from build123d import *

# Parameters (mm, degrees)
BOSS_EXTRUDE1_DEPTH = 64.15
SKETCH2_R           = 1.75
CUT_EXTRUDE1_DEPTH  = 2.42
CUT_EXTRUDE2_DEPTH  = 2.42
SKETCH4_R           = 1.54
CUT_EXTRUDE3_DEPTH  = 2.42


with BuildPart() as part:
    # Sketch1 → Boss-Extrude1 (new, symmetric)
    with BuildSketch(Plane(origin=(0, 0, 0), x_dir=(0, 0, -1), z_dir=(1, 0, 0))):
        with BuildLine():
            Line((-22.947001366, 0), (-3.987001366, 0))
            ThreePointArc((-3.987001366, 0), (-1.844787094, 1.175258995), (-1.684979587, 3.613450385))
            Line((-1.684979587, 3.613450385), (-7.115854863, 15.26))
            Line((-7.115854863, 15.26), (-9.309119708, 14.237263807))
            Line((-9.309119708, 14.237263807), (-3.878244431, 2.590714191))
            ThreePointArc((-3.878244431, 2.590714191), (-3.885794392, 2.475524047), (-3.987001366, 2.42))
            Line((-3.987001366, 2.42), (-22.947001366, 2.42))
            Line((-22.947001366, 2.42), (-22.947001366, 0))
        make_face()
    extrude(amount=BOSS_EXTRUDE1_DEPTH, both=True)

    # Sketch2 → Cut-Extrude1 (cut)
    with BuildSketch(Plane(origin=(0, 0, 0), x_dir=(-1, 0, 0), z_dir=(0, 0.4226182617407038, -0.9063077870366478))):
        with BuildLine():
            ThreePointArc((-64.15, 11.687547043), (-62.641599916, 15.329146974), (-58.999999979, 16.837547043))
            Line((-58.999999979, 16.837547043), (-64.15, 16.837547043))
            Line((-64.15, 16.837547043), (-64.15, 11.687547043))
        make_face()
        with BuildLine():
            ThreePointArc((54.05757399, 13.134932664), (55.912244813, 15.809229698), (58.999999973, 16.837547043))
            Line((58.999999973, 16.837547043), (-58.999999979, 16.837547043))
            ThreePointArc((-58.999999979, 16.837547043), (-55.912244816, 15.8092297), (-54.05757399, 13.134932664))
            ThreePointArc((-54.05757399, 13.134932664), (-53.157248342, 11.836730217), (-51.658338063, 11.337547043))
            Line((-51.658338063, 11.337547043), (51.658338063, 11.337547043))
            ThreePointArc((51.658338063, 11.337547043), (53.157248342, 11.836730217), (54.05757399, 13.134932664))
        make_face()
        with BuildLine():
            ThreePointArc((58.999999973, 16.837547043), (62.641599913, 15.329146976), (64.15, 11.687547043))
            Line((64.15, 11.687547043), (64.15, 16.837547043))
            Line((64.15, 16.837547043), (58.999999973, 16.837547043))
        make_face()
        with Locations(Location((-59, 11.687547043, 0), (0, 0, 90))):
            Circle(SKETCH2_R)
        with Locations(Location((59, 11.687547043, 0), (0, 0, 90))):
            Circle(SKETCH2_R)
    extrude(amount=-CUT_EXTRUDE1_DEPTH, mode=Mode.SUBTRACT)

    # Sketch3 → Cut-Extrude2 (cut)
    with BuildSketch(Plane.XZ):
        with BuildLine():
            ThreePointArc((-64.15, 4.347001366), (-62.451219331, 8.448220697), (-58.35, 10.147001366))
            Line((-58.35, 10.147001366), (-49, 10.147001366))
            Line((-49, 10.147001366), (-27.188464844, 22.394753573))
            ThreePointArc((-27.188464844, 22.394753573), (-23.20933914, 22.359091991), (-21.23, 18.907001366))
            Line((-21.23, 18.907001366), (-21.23, 15.907001366))
            ThreePointArc((-21.23, 15.907001366), (-20.937106781, 15.199894585), (-20.23, 14.907001366))
            Line((-20.23, 14.907001366), (20.23, 14.907001366))
            ThreePointArc((20.23, 14.907001366), (20.937106781, 15.199894585), (21.23, 15.907001366))
            Line((21.23, 15.907001366), (21.23, 18.907001366))
            ThreePointArc((21.23, 18.907001366), (23.20933914, 22.359091991), (27.188464844, 22.394753573))
            Line((27.188464844, 22.394753573), (49, 10.147001366))
            Line((49, 10.147001366), (58.35, 10.147001366))
            ThreePointArc((58.35, 10.147001366), (62.451219331, 8.448220697), (64.15, 4.347001366))
            Line((64.15, 4.347001366), (64.15, 22.947001366))
            Line((64.15, 22.947001366), (-64.15, 22.947001366))
            Line((-64.15, 22.947001366), (-64.15, 4.347001366))
        make_face()
    extrude(amount=-CUT_EXTRUDE2_DEPTH, mode=Mode.SUBTRACT)

    # Sketch4 → Cut-Extrude3 (cut)
    with BuildSketch(Plane.XZ):
        with Locations(Location((-25.23, 18.907001366, 0), (0, 0, 270))):
            Circle(SKETCH4_R)
        with Locations(Location((-30, 16.228520571, 0), (0, 0, 270))):
            Circle(SKETCH4_R)
        with Locations(Location((-34.77, 13.550039776, 0), (0, 0, 270))):
            Circle(SKETCH4_R)
        with Locations(Location((-31.275605409, 11.933962289, 0), (0, 0, 270))):
            Circle(SKETCH4_R)
        with Locations(Location((-39.521703084, 11.753454736, 0), (0, 0, 270))):
            Circle(SKETCH4_R)
        with Locations(Location((-44.354096024, 10.186809126, 0), (0, 0, 270))):
            Circle(SKETCH4_R)
        with Locations(Location((-26.498719925, 8.557001366, 0), (0, 0, 270))):
            Circle(SKETCH4_R)
    cut_extrude3 = extrude(amount=-CUT_EXTRUDE3_DEPTH, mode=Mode.SUBTRACT)

    # Mirror1: Cut-Extrude3 across plane
    add(cut_extrude3.mirror(Plane(origin=(0, 0, 0), x_dir=(0, 0, 1), z_dir=(1, 0, 0))), mode=Mode.SUBTRACT)


solid = part.part
Input: part model. Units: mm. Frame: model coordinates. A direction names the side the tool comes from. Round coordinates to 2 decimals unless told otherwise and drop trailing zeros. Order: outer loops, then holes, each group sorted by start corner. A loop starts at its lowest first (then second) coordinate and runs counter-clockwise, first axis right, second up. Notation, with made-up numbers: (56, 28.5) - (74, 28.5) arc R33 ccw to (74, 59.5) - close; hole circle Ø7 at (12, 16). An arc over 180 degrees is marked (long way). Answer as a JSON object with one key per item and string values. Group by question number.
(1) Reachability of faces 5 (the face through (-54, 1, 10.147)), 6 (the face through (1, 2.42, 9)), 7 (the face through (54, 1, 10.147)), 8 (the face through (62.4, 1.2, 8.5)) from +Z, -Z, +X, -X, +Y, -Y: full face, straight path, thin tool, end or side. Return the list, or none.
(2) Cut plane A-A (x = 9.5). Return loops of the section in (y, z).
(3) Draft query along Z for faces 1 (the face through (-29.932, 1.193, 17.767)), 2 (the face through (37.942, 1.193, 16.357)), 3 (the face through (64.15, 5, 4)), 4 (the face through (0.9, 8.06, 3.76)). Return one class per face: released by +Z, released by -Z, zero draft, split by the parting line, or undercut.
(4) Pin query (flat end, axial travel): P1, Ø5.5, axis at x = 24.5, z = 9.5, coming from the +Y side; P2, Ø1.9, axis at x = 53.5, y = 1, coming from the +Z side; P3, Ø2, axis at x = 2.5, z = 16.5, coming from the -Y side; P4, Ø2.5, axis at x = 2, y = 1.5, coming from the +Z side. Return the tip coordinate at first contact, or that it passes through.
(5) Cut plane C-C (x = -53). Return loops of the section in (y, z), then the cut area to 3 significant figures.
(6) Material intervals for probe 1 along Z at (x, y) = (30, 0.75); probe 2 along Y at (x, z) = (17, 7.75); probe 3 along X at (y, z) = (2.25, 21), sorted ascending. Write a range as from..to.
(7) Cut plane B-B (x = -34.77). Return loops of the section in (y, z), then the cut area to 3 significant figures.
Here are the results:
{
 "1": {"face 5": "+Z, -X, +Y, -Y", "face 6": "+Z, +X, -X", "face 7": "+Z, +X, +Y, -Y", "face 8": "+Z, +X, -Y"},
 "2": {"outline": "(0, 3.99) arc R2.54 ccw to (3.61, 1.68) - (10.28, 4.79) - (9.25, 6.98) - (2.59, 3.88) arc R0.12 cw to (2.42, 3.99) - (2.42, 14.91) - (0, 14.91) - close"},
 "3": {"face 1": "undercut", "face 2": "released by +Z", "face 3": "zero draft", "face 4": "released by -Z"},
 "4": {"P1": "stops at y = 9.36", "P2": "stops at z = 10.15", "P3": "passes through", "P4": "stops at z = 14.91"},
 "5": {"outline": "(0, 3.99) arc R2.54 ccw to (3.61, 1.68) - (10.63, 4.96) - (9.61, 7.15) - (2.59, 3.88) arc R0.12 cw to (2.42, 3.99) - (2.42, 10.15) - (0, 10.15) - close", "area": "40.1 mm^2"},
 "6": {"probe 1": "z = 2.18..11.07, 12.8..14.69, 17.77..20.82", "probe 2": "y = 0..2.42", "probe 3": "x = -29.67..-21.82, 21.82..29.67"},
 "7": {"outline": "(0, 3.99) arc R2.54 ccw to (3.61, 1.68) - (10.28, 4.79) - (9.25, 6.98) - (2.59, 3.88) arc R0.12 cw to (2.42, 3.99) - (2.42, 12.01) - (0, 12.01) - close; (0, 15.09) - (2.42, 15.09) - (2.42, 18.14) - (0, 18.14) - close", "area": "51.0 mm^2"}
}
